Part print with two shaded views. Sizes in mm from the minimum x, y, z corner. Give positions to 0.01 mm unless a question says otherwise; leave off trailing zeros. Write each loop counter-clockwise with the first axis right and the second up, starting at its lowest first coordinate (ties: lowest second). Pieces come first, ordered by that corner, then holes.
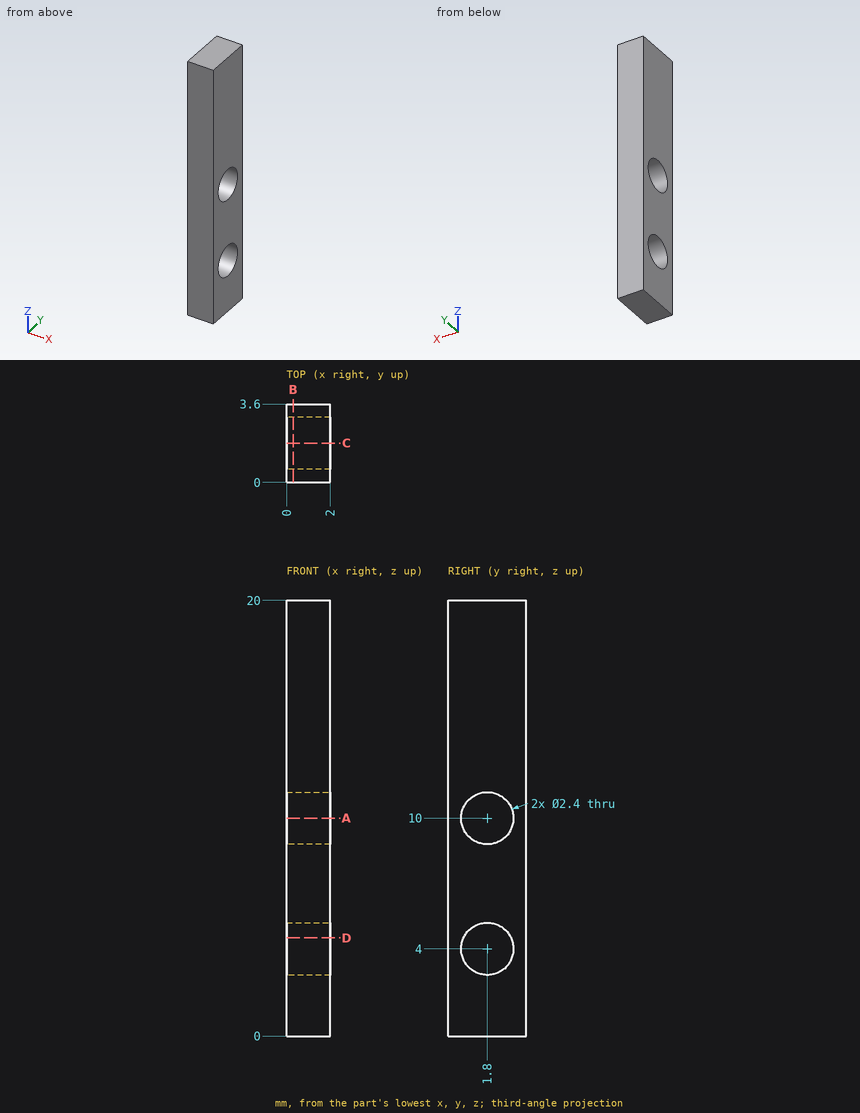
1) Wall check: L1, parallel to Z at x = 1.8, y = 1.7; L2, parallel to Y at x = 0.95, z = 10; L3, parallel to Z at x = 0.9, y = 2.5. Give the ranges that are in metal, low to high.
Answers follow:
L1: z = 0 to 2.8, 5.2 to 8.8, 11.2 to 20
L2: y = 0 to 0.6, 3 to 3.6
L3: z = 0 to 3.03, 4.97 to 9.03, 10.97 to 20
2) Saw through at B-B, the plane x = 0.3. Write the cut outline in (y, z).
Answers follow:
outline: (0, 0) - (3.6, 0) - (3.6, 20) - (0, 20) - close; hole circle Ø2.4 at (1.8, 4); hole circle Ø2.4 at (1.8, 10)
3) Saw through at D-D, the plane z = 4.5. Write the cut outline in (x, y), then the cut area to 3 significant figures.
Answers follow:
outline: (0, 0) - (2, 0) - (2, 0.71) - (0, 0.71) - close; (0, 2.89) - (2, 2.89) - (2, 3.6) - (0, 3.6) - close
area: 2.84 mm2
4) Saw through at A-A, the plane z = 10. Write the cut outline in (x, y), then the cut area to 3 significant figures.
Answers follow:
outline: (0, 0) - (2, 0) - (2, 0.6) - (0, 0.6) - close; (0, 3) - (2, 3) - (2, 3.6) - (0, 3.6) - close
area: 2.40 mm2
5) Saw through at C-C, the plane y = 1.8. Write the cut outline in (x, z), then the cut area to 3 significant figures.
Answers follow:
outline: (0, 0) - (2, 0) - (2, 2.8) - (0, 2.8) - close; (0, 5.2) - (2, 5.2) - (2, 8.8) - (0, 8.8) - close; (0, 11.2) - (2, 11.2) - (2, 20) - (0, 20) - close
area: 30.4 mm2
